Part model, mm, in its own coordinate system. Face numbers are marked on the shaded views. A direction names the side the tool comes from. Give positions to 0.01 mm unless a question says otherwise; leave off trailing zeros. Order: outer loops, then holes, each group sorted by start corner. A loop starts at its lowest first (then second) coordinate and runs counter-clockwise, first axis right, second up. Notation, with made-up numbers: (59.5, -12) - (103.5, -12) arc R19 cw to (103.5, 6) - close; hole circle Ø9 at (-16.75, 20.25). An arc over 180 degrees is marked (long way). Use a Markdown table: item, result. Add a question column.
from build123d import *

# Parameters (mm, degrees)
BOSS_EXTRUDE1_DEPTH = 10
CUT_EXTRUDE1_REACH  = 80.74
SKETCH2_W           = 35
SKETCH2_H           = 5
CUT_EXTRUDE2_REACH  = 61.161
SKETCH3_R           = 7
BOSS_EXTRUDE2_DEPTH = 22
CUT_EXTRUDE3_DEPTH  = 22


with BuildPart() as part:
    # Sketch1 → Boss-Extrude1 (new body)
    with BuildSketch(Plane.XY):
        with BuildLine():
            Line((-35, 30), (35, 30))
            ThreePointArc((35, 30), (45.606601718, 25.606601718), (50, 15))
            Line((50, 15), (50, -15))
            ThreePointArc((50, -15), (45.606601718, -25.606601718), (35, -30))
            Line((35, -30), (-35, -30))
            ThreePointArc((-35, -30), (-45.606601718, -25.606601718), (-50, -15))
            Line((-50, -15), (-50, 15))
            ThreePointArc((-50, 15), (-45.606601718, 25.606601718), (-35, 30))
        make_face()
    extrude(amount=BOSS_EXTRUDE1_DEPTH)

    # Sketch2 → Cut-Extrude1 (cut, up to next)
    with BuildSketch(Plane.XZ.offset(30), mode=Mode.PRIVATE) as cut_extrude1_sk1:
        with Locations((0, 2.5)):
            Rectangle(SKETCH2_W, SKETCH2_H)
    cut_extrude1_tool1 = extrude(cut_extrude1_sk1.sketch, amount=-CUT_EXTRUDE1_REACH, mode=Mode.PRIVATE) & part.part
    add(cut_extrude1_tool1.solids().sort_by_distance((0, -30, 2.5))[0], mode=Mode.SUBTRACT)

    # Sketch3 → Cut-Extrude2 (cut, up to next)
    with BuildSketch(Plane.XY.offset(10), mode=Mode.PRIVATE) as cut_extrude2_sk1:
        with Locations((-35, 15)):
            Circle(SKETCH3_R)
    cut_extrude2_tool1 = extrude(cut_extrude2_sk1.sketch, amount=-CUT_EXTRUDE2_REACH, mode=Mode.PRIVATE) & part.part
    # Sketch3 → Cut-Extrude2 (cut, up to next)
    with BuildSketch(Plane.XY.offset(10), mode=Mode.PRIVATE) as cut_extrude2_sk2:
        with Locations((35, 15)):
            Circle(SKETCH3_R)
    cut_extrude2_tool2 = extrude(cut_extrude2_sk2.sketch, amount=-CUT_EXTRUDE2_REACH, mode=Mode.PRIVATE) & part.part
    # Sketch3 → Cut-Extrude2 (cut, up to next)
    with BuildSketch(Plane.XY.offset(10), mode=Mode.PRIVATE) as cut_extrude2_sk3:
        with Locations((35, -15)):
            Circle(SKETCH3_R)
    cut_extrude2_tool3 = extrude(cut_extrude2_sk3.sketch, amount=-CUT_EXTRUDE2_REACH, mode=Mode.PRIVATE) & part.part
    # Sketch3 → Cut-Extrude2 (cut, up to next)
    with BuildSketch(Plane.XY.offset(10), mode=Mode.PRIVATE) as cut_extrude2_sk4:
        with Locations((-35, -15)):
            Circle(SKETCH3_R)
    cut_extrude2_tool4 = extrude(cut_extrude2_sk4.sketch, amount=-CUT_EXTRUDE2_REACH, mode=Mode.PRIVATE) & part.part
    add(cut_extrude2_tool1.solids().sort_by_distance((-35, 15, 10))[0], mode=Mode.SUBTRACT)
    add(cut_extrude2_tool2.solids().sort_by_distance((35, 15, 10))[0], mode=Mode.SUBTRACT)
    add(cut_extrude2_tool3.solids().sort_by_distance((35, -15, 10))[0], mode=Mode.SUBTRACT)
    add(cut_extrude2_tool4.solids().sort_by_distance((-35, -15, 10))[0], mode=Mode.SUBTRACT)

    # Sketch4 → Boss-Extrude2 (add)
    with BuildSketch(Plane.XY.offset(10)):
        with BuildLine():
            Line((-10, 12), (10, 12))
            ThreePointArc((10, 12), (22, 0), (10, -12))
            Line((10, -12), (-10, -12))
            ThreePointArc((-10, -12), (-22, 0), (-10, 12))
        make_face()
    extrude(amount=BOSS_EXTRUDE2_DEPTH)

    # Sketch5 → Cut-Extrude3 (cut)
    with BuildSketch(Plane.XY.offset(32)):
        with BuildLine():
            Line((-10, 8), (10, 8))
            ThreePointArc((10, 8), (18, 0), (10, -8))
            Line((10, -8), (-10, -8))
            ThreePointArc((-10, -8), (-18, 0), (-10, 8))
        make_face()
    extrude(amount=-CUT_EXTRUDE3_DEPTH, mode=Mode.SUBTRACT)


solid = part.part
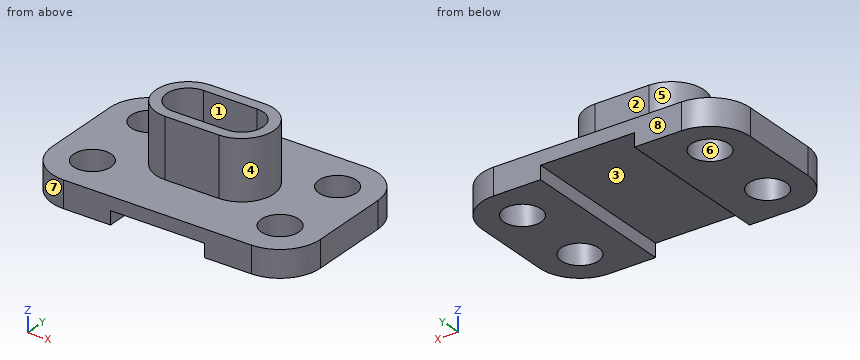
1. Cut at A-A (z = 22). Write the cut outline in (x, y), plus the area to 3 significant figures.
2. Drill centre lines: probe 1 along Y at (x, z) = (35, 2); probe 2 along Z at (x, y) = (3, 12.5); probe 3 along Z at (x, y) = (18, 25.5). Where is each one in solid material? Low to high. Write a range as [from, to].
3. Tool access for the marked faces 1, 2, 3, 4 and 5: list every direction of +Z, -Z, +X, -X, +Y, -Y with a clear straight run to the whole face (end or side of a thin tool).
4. Cut at D-D (x = -30). Write the cut outline in (y, z).
5. Mould opens along X. For the marked faces 6, 7 and 8 say: released by +X, released by -X, zero draft, split by the parting line, or undercut.
6. Cut at B-B (z = 7). Write the cut outline in (x, y).
7. Pin check, flat tips, straight feed: P1, Ø6, axis at x = 0, z = 24.5, coming from the +Y side; P2, Ø2, axis at x = 15, y = 13.5, coming from the +Z side; P3, Ø16, axis at x = 0, z = 22, coming from the -Y side; P4, Ø3, axis at y = 18.5, z = 13, coming from the +X side. Stop position of each tip, or through.
8. Cut at C-C (y = -9.5). Write the cut outline in (x, z).
Responses:
| question | item | result |
|---|---|---|
| 1 | outline | (-10, -12) - (10, -12) arc R12 ccw to (10, 12) - (-10, 12) arc R12 ccw to start; hole (-10, -8) - (10, -8) arc R8 ccw to (10, 8) - (-10, 8) arc R8 ccw to start |
| 1 | area | 411 mm² |
| 2 | probe 1 | y = [-30, -22], [-8, 8], [22, 30] |
| 2 | probe 2 | z = [5, 10] |
| 2 | probe 3 | z = [0, 10] |
| 3 | face 1 | +Z |
| 3 | face 2 | +Z, +X, -X, +Y |
| 3 | face 3 | -Z, +Y, -Y |
| 3 | face 4 | +Z, +X |
| 3 | face 5 | +Z, -X |
| 4 | outline | (-30, 0) - (-19.9, 0) - (-19.9, 10) - (-30, 10) - close; (-10.1, 0) - (10.1, 0) - (10.1, 10) - (-10.1, 10) - close; (19.9, 0) - (30, 0) - (30, 10) - (19.9, 10) - close |
| 5 | face 6 | undercut |
| 5 | face 7 | released by -X |
| 5 | face 8 | zero draft |
| 6 | outline | (-50, -15) arc R15 ccw to (-35, -30) - (35, -30) arc R15 ccw to (50, -15) - (50, 15) arc R15 ccw to (35, 30) - (-35, 30) arc R15 ccw to (-50, 15) - close; hole circle Ø14 at (-35, -15); hole circle Ø14 at (-35, 15); hole circle Ø14 at (35, -15); hole circle Ø14 at (35, 15) |
| 7 | P1 | stops at y = 12 |
| 7 | P2 | stops at z = 10 |
| 7 | P3 | stops at y = -12 |
| 7 | P4 | passes through |
| 8 | outline | (-50, 0) - (-39.33, 0) - (-39.33, 10) - (-50, 10) - close; (-30.67, 0) - (-17.5, 0) - (-17.5, 5) - (17.5, 5) - (17.5, 0) - (30.67, 0) - (30.67, 10) - (17.33, 10) - (17.33, 32) - (-17.33, 32) - (-17.33, 10) - (-30.67, 10) - close; (39.33, 0) - (50, 0) - (50, 10) - (39.33, 10) - close |
